Work out the finished part from the listing and answer in its coordinate system (mm). A direction names the side the tool comes from. Give positions to 0.01 mm unless a question says otherwise; leave off trailing zeros. Loops run counter-clockwise (first coordinate to the right, second up) from the corner with the lowest first, then second, coordinate; pieces in that order, holes last. Notation, with made-up numbers: (-1, -28) - (27, -28) arc R22 ccw to (27, -18) - close; hole circle Ø6 at (85.25, -39.75). An arc over 180 degrees is marked (long way). One line per question, with ' | ' between items.
from build123d import *

# Parameters (mm, degrees)
SKETCH_3_R          = 1.5
CUT_EXTRUDE_1_DEPTH = 84.821641
SKETCH_2_R          = 51.5
SKETCH_2_W          = 56
SKETCH_2_H          = 72
EXTRUDE_1_DEPTH     = 3
SKETCH_4_R          = 1
SKETCH_4_R_2        = 2.5
EXTRUDE_2_DEPTH     = 2
SKETCH_5_R          = 1.2
CUT_EXTRUDE_2_DEPTH = 84.800029833
FILLET_2_R          = 3
SKETCH_11_R         = 1.5
CUT_EXTRUDE_6_DEPTH = 84.821641


with BuildPart() as part:
    # 草图1 → 旋转1 (revolve)
    with BuildSketch(Plane.XY, mode=Mode.PRIVATE) as revolve_1_sk:
        Polygon((51.5, 2.35), (51.5, -3), (59.15, -3), (59.15, 0), (57.15, 0), (57.15, 2.35), align=None)
    revolve(revolve_1_sk.sketch.rotate(Axis((0, 0, 0), (0, 1, 0)), 90), axis=Axis((0, 0, 0), (0, 1, 0)))

    # 草图3 → 切除-拉伸1 (cut, through all)
    with BuildSketch(Plane(origin=(0, 2.35, 0), x_dir=(1, 0, 0), z_dir=(0, 1, 0))):
        with Locations(Location((-16.5, -51.942275653, 0), (0, 0, 270))):
            Circle(SKETCH_3_R)
        with Locations(Location((-22.5, -49.638694584, 0), (0, 0, 270))):
            Circle(SKETCH_3_R)
        with Locations(Location((-22.5, 49.638694584, 0), (0, 0, 90))):
            Circle(SKETCH_3_R)
        with Locations(Location((-16.5, 51.942275653, 0), (0, 0, 90))):
            Circle(SKETCH_3_R)
        with Locations(Location((16.5, 51.942275653, 0), (0, 0, 270))):
            Circle(SKETCH_3_R)
        with Locations(Location((22.5, 49.638694584, 0), (0, 0, 270))):
            Circle(SKETCH_3_R)
        with Locations(Location((22.5, -49.638694584, 0), (0, 0, 90))):
            Circle(SKETCH_3_R)
        with Locations(Location((16.5, -51.942275653, 0), (0, 0, 90))):
            Circle(SKETCH_3_R)
    extrude(amount=-CUT_EXTRUDE_1_DEPTH, mode=Mode.SUBTRACT)

    # 草图2 → 凸台-拉伸1 (add)
    with BuildSketch(Plane.XZ.offset(3)):
        with Locations(Location((0, 0, 0), (0, 0, 270))):
            Circle(SKETCH_2_R)
        Rectangle(SKETCH_2_W, SKETCH_2_H, mode=Mode.SUBTRACT)
    extrude(amount=-EXTRUDE_1_DEPTH)

    # 草图4 → 凸台-拉伸2 (add)
    with BuildSketch(Plane(origin=(0, 0, 0), x_dir=(1, 0, 0), z_dir=(0, 1, 0))):
        with Locations(Location((31, -13, 0), (0, 0, 90))):
            Circle(SKETCH_4_R)
        with Locations(Location((-31, -13, 0), (0, 0, 90))):
            Circle(SKETCH_4_R)
        with Locations(Location((-31, 13, 0), (0, 0, 90))):
            Circle(SKETCH_4_R)
        with Locations(Location((31, 13, 0), (0, 0, 90))):
            Circle(SKETCH_4_R)
        with Locations(Location((31, 0, 0), (0, 0, 90))):
            Circle(SKETCH_4_R_2)
        with Locations(Location((-31, 0, 0), (0, 0, 90))):
            Circle(SKETCH_4_R_2)
    extrude(amount=EXTRUDE_2_DEPTH)

    # 草图5 → 切除-拉伸2 (cut, through all)
    with BuildSketch(Plane(origin=(0, 2, 0), x_dir=(1, 0, 0), z_dir=(0, 1, 0))):
        with Locations(Location((31, 0, 0), (0, 0, 270))):
            Circle(SKETCH_5_R)
        with Locations(Location((-31, 0, 0), (0, 0, 270))):
            Circle(SKETCH_5_R)
    extrude(amount=-CUT_EXTRUDE_2_DEPTH, mode=Mode.SUBTRACT)

    # 圆角2
    fillet_2_edges = [part.edges().sort_by_distance(p)[0] for p in [
        (-28, -1.5, -36),
        (28, -1.5, -36),
        (28, -1.5, 36),
        (-28, -1.5, 36),
    ]]
    fillet(fillet_2_edges, radius=FILLET_2_R)

    # 草图11 → 切除-拉伸6 (cut, through all)
    with BuildSketch(Plane.XZ.offset(3)):
        with Locations(Location((-53.047148839, 12.5, 0), (0, 0, 270))):
            Circle(SKETCH_11_R)
        with Locations(Location((53.047148839, 12.5, 0), (0, 0, 90))):
            Circle(SKETCH_11_R)
        with Locations(Location((53.047148839, -12.5, 0), (0, 0, 270))):
            Circle(SKETCH_11_R)
        with Locations(Location((-53.047148839, -12.5, 0), (0, 0, 90))):
            Circle(SKETCH_11_R)
    extrude(amount=-CUT_EXTRUDE_6_DEPTH, mode=Mode.SUBTRACT)


solid = part.part
1. Which of the six approach directions +Z, -Z, +X, -X, +Y, -Y give full straight-line access (tool end or side, diameter ignored) to faces 1 (the flat face through (30, 2, -1)), 2 (the flat face through (0, -2, 36))?
Evaluation:
face 1: +Y | face 2: +Y, -Y
2. Consider L1, parallel to X at y = -0.8, z = 0; L2, parallel to Z at x = 29, y = 1.95; L3, parallel to Z at x = -23, y = 0.8. Determine where each line is inside the solid, lowest interval first.
Evaluation:
L1: -59.15 to -32.2, -29.8 to -28, 28 to 29.8, 32.2 to 59.15 | L2: -49.25 to -42.56, -1.5 to 1.5, 42.56 to 49.25 | L3: -52.32 to -51.05, -48.22 to -46.08, 46.08 to 48.22, 51.05 to 52.32
3. Find section A-A on x = -16.5. Write down the section's boundary in (y, z), then the cut area to 3 significant figures.
Evaluation:
outline: (-3, -56.8) - (0, -56.8) - (0, -54.72) - (2.35, -54.72) - (2.35, -53.44) - (-3, -53.44) - close; (-3, -50.44) - (2.35, -50.44) - (2.35, -48.79) - (0, -48.79) - (0, -36) - (-3, -36) - close; (-3, 36) - (0, 36) - (0, 48.79) - (2.35, 48.79) - (2.35, 50.44) - (-3, 50.44) - close; (-3, 53.44) - (2.35, 53.44) - (2.35, 54.72) - (0, 54.72) - (0, 56.8) - (-3, 56.8) - close | area: 121 mm2
4. Find section D-D on z = 41. Write down the section's boundary in (x, y).
Evaluation:
outline: (-42.63, -3) - (42.63, -3) - (42.63, 0) - (39.81, 0) - (39.81, 2.35) - (31.16, 2.35) - (31.16, 0) - (-31.16, 0) - (-31.16, 2.35) - (-39.81, 2.35) - (-39.81, 0) - (-42.63, 0) - close
5. Flat-ended cylindrical pins translate along their axes: pin 1 (2.5 mm diameter, centred on x = 6, y = -1, fed in from +Z); pin 2 (1.5 mm diameter, centred on y = 1, z = -18, fed in from +X); pin 3 (2 mm diameter, centred on x = 32.5, z = 6.5, fed in from +Y). Find the tip coordinate at first contact, or state that the pin passes through.
Evaluation:
pin 1: z = 58.96 | pin 2: x = 54.48 | pin 3: y = 0
6. Find section B-B on z = -23.5. Write down the section's boundary in (x, y).
Evaluation:
outline: (-54.28, -3) - (-28, -3) - (-28, 0) - (-45.83, 0) - (-45.83, 2.35) - (-52.09, 2.35) - (-52.09, 0) - (-54.28, 0) - close; (28, -3) - (54.28, -3) - (54.28, 0) - (52.09, 0) - (52.09, 2.35) - (45.83, 2.35) - (45.83, 0) - (28, 0) - close
7. Determine the mould class of faces 3 (the flat face through (-48.5, 0, 30.9)), 4 (the cylindrical face through (-54.51, -0.36, 12.83)), 5 (the cylindrical face through (-17.767, -1.479, -56.419)) for opening direction X: +X half, -X half, draft (parallel to the pull), parting line (faces both ways), or undercut.
Evaluation:
face 3: draft | face 4: undercut | face 5: parting line
8. Find section C-C on y = -1.2. State how many separate pieces and enclosed holes the cut face has, then the cut area to 3 significant figures.
Evaluation:
separate pieces: 1 | enclosed holes: 15 | area: 6,870 mm2
